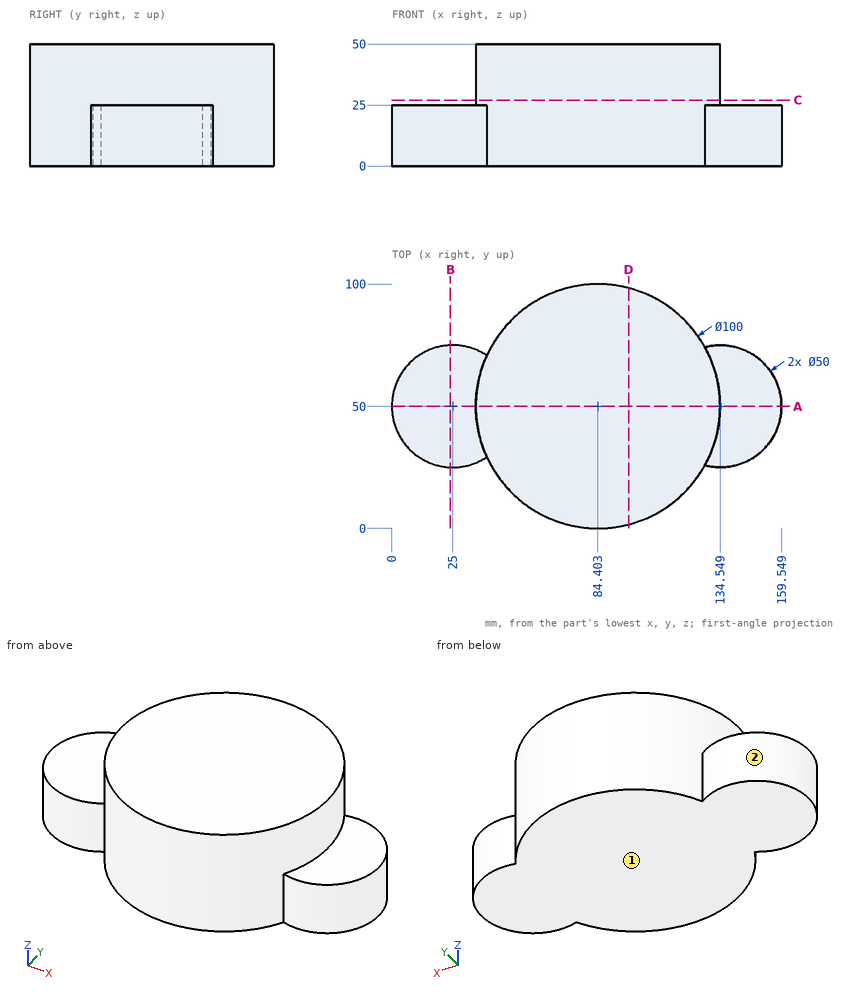
The figure shows three views and two pictorial views of one solid part (mm, origin at its lowest corner). Answer the questions. Give positions to 0.01 mm unless a question says otherwise; leave off trailing zeros. Write each loop counter-clockwise with the first axis right and the second up, starting at its lowest first coordinate (ties: lowest second). Pieces come first, ordered by that corner, then holes. Notation, with made-up numbers: (63, 70.25) - (102, 70.25) arc R14 ccw to (102, 91.25) - close; hole circle Ø1 at (52, -13.5). An arc over 180 degrees is marked (long way). Return JSON: item names as keys, results as strings.
Q1. A cutting plane is placed at C-C, the plane z = 27. Determine the outline of the cut face in (x, y).
Reply:
{"outline": "circle Ø100 at (84.4, 50)"}
Q2. A cutting plane is placed at B-B, the plane x = 24. Determine the outline of the cut face in (y, z), and give its area (3 significant figures).
Reply:
{"outline": "(25.02, 0) - (74.98, 0) - (74.98, 25) - (25.02, 25) - close", "area": "1,250 mm²"}
Q3. A cutting plane is placed at D-D, the plane x = 97. Determine the outline of the cut face in (y, z).
Reply:
{"outline": "(1.61, 0) - (98.39, 0) - (98.39, 50) - (1.61, 50) - close"}
Q4. Consider line 1 along Y through (x, z) = (85, 29.5); line 2 along Y through (x, z) = (27.5, 19) (1 decimal); line 3 along X through (y, z) = (19, 38.5) (1 decimal). Determine where each line is inside the solid, lowest interval first. Write a range as [from, to].
Reply:
{"line 1": "[0, 100]", "line 2": "[25.1, 74.9]", "line 3": "[45.2, 123.6]"}
Q5. Given P1, Ø9.5, axis at x = 140, y = 38, coming from the +Z side; P2, Ø6, axis at y = 23.5, z = 33.5, coming from the -X side; P3, Ø8, axis at y = 66.5, z = 39.5, coming from the +X side (1 decimal); P4, Ø4, axis at x = 117.5, y = 77.5, coming from the -Z side, each flat-ended and moving along its own axis, determine where each tip first touches the part or whether it passes through.
Reply:
{"P1": "z = 25", "P2": "x = 40.27", "P3": "x = 132.8", "P4": "z = 0"}
Q6. For a pull along X with two mould halves and no side action, classify the marked faces 1 and 2 as released by +X, released by -X, zero draft, split by the parting line, or undercut.
Reply:
{"face 1": "zero draft", "face 2": "undercut"}
Q7. A cutting plane is placed at A-A, the plane y = 50. Determine the outline of the cut face in (x, z).
Reply:
{"outline": "(0, 0) - (159.55, 0) - (159.55, 25) - (134.4, 25) - (134.4, 50) - (34.4, 50) - (34.4, 25) - (0, 25) - close"}
